Could you check a few things on this model? Use its own coordinates, in mm. A direction names the side the tool comes from. Give positions to 0.01 mm unless a question says otherwise; leave off trailing zeros. Loops run counter-clockwise (first coordinate to the right, second up) from the corner with the lowest first, then second, coordinate; pieces in that order, holes last. Notation, with made-up numbers: M -32.75,60 L -11.75,60 A26 ccw -11.75,94 Z; hole C 12,-11 d8. An arc over 180 degrees is marked long. Use a Markdown table: item, result. Add a question column.
1) Which directions (+Z, -Z, +X, -X, +Y, -Y) give clear straight access to the entire face, cutting with the end or side of a thin tool? Please do faces 1 (the cylindrical face through (190.979, -81.445, 2.535)), 2 (the cylindrical face through (131.071, -57.995, 2.465)).
2) We'd pull the mould along Y, two halves only. Please class faces 3 (the flat face through (121, -64, 0)), 4 (the cylindrical face through (8.555, -80.979, 2.535)), 5 (the flat face through (70, -72, 2)): +Y half, -Y half, draft (parallel to the pull), parting line (faces both ways), or undercut.
3) If I drill on line 1 along Y through (x, z) = (109, 2.15); line 2 along Y through (x, z) = (185, 2.5); line 3 along Y through (x, z) = (51, 1.6), over which ranges is the centre line in solid material (lowest first)? Write a range as [from, to].
4) Suppose I cut it at A-A on x = 131.5. List the corners of the cut face in (y, z) for me.
5) Suppose I cut it at D-D on y = -82.5. List the corners of the cut face in (x, z) for me.
6) Suppose I cut it at B-B on z = 2.55. Count the separate pieces of the cut face and the enclosed holes in it, and give its area (3 significant figures).
7) Suppose I cut it at C-C on x = 81. List the corners of the cut face in (y, z) for me.
```python
from build123d import *

# Parameters (mm, degrees)
SKETCH_W    = 200
SKETCH_H    = 90
SKETCH_R    = 1.5625
SKETCH_W_2  = 60
SKETCH_H_2  = 67
PAD_DEPTH   = 5
FILLET_R    = 30
FILLET001_R = 3.125
FILLET002_R = 1


with BuildPart() as part:
    # Sketch → Pad (new body)
    with BuildSketch(Plane.XY):
        with Locations((100, -45)):
            Rectangle(SKETCH_W, SKETCH_H)
        with Locations((175, -10)):
            Circle(SKETCH_R, mode=Mode.SUBTRACT)
        with Locations((175, -30)):
            Circle(SKETCH_R, mode=Mode.SUBTRACT)
        with Locations((185, -20)):
            Circle(SKETCH_R, mode=Mode.SUBTRACT)
        with Locations((185, -40)):
            Circle(SKETCH_R, mode=Mode.SUBTRACT)
        with Locations((25, -10)):
            Circle(SKETCH_R, mode=Mode.SUBTRACT)
        with Locations((25, -30)):
            Circle(SKETCH_R, mode=Mode.SUBTRACT)
        with Locations((15, -20)):
            Circle(SKETCH_R, mode=Mode.SUBTRACT)
        with Locations((15, -40)):
            Circle(SKETCH_R, mode=Mode.SUBTRACT)
        with Locations((70, -38.5)):
            Rectangle(SKETCH_W_2, SKETCH_H_2, mode=Mode.SUBTRACT)
        with BuildLine():
            ThreePointArc((158.0113, -4.9887), (155.0113, -1.9887), (152.0113, -4.9887))
            Line((152.0113, -4.9887), (152.0113, -14.9887))
            ThreePointArc((152.0113, -14.9887), (155.0113, -17.9887), (158.0113, -14.9887))
            Line((158.0113, -4.9887), (158.0113, -14.9887))
        make_face(mode=Mode.SUBTRACT)
        with BuildLine():
            ThreePointArc((151, -28.5), (131.5, -9), (112, -28.5))
            Line((112, -28.5), (112, -38.5))
            ThreePointArc((112, -38.5), (131.5, -58), (151, -38.5))
            Line((151, -28.5), (151, -38.5))
        make_face(mode=Mode.SUBTRACT)
        with BuildLine():
            ThreePointArc((158.0113, -52.0113), (155.0113, -49.0113), (152.0113, -52.0113))
            Line((152.0113, -52.0113), (152.0113, -62.0113))
            ThreePointArc((152.0113, -62.0113), (155.0113, -65.0113), (158.0113, -62.0113))
            Line((158.0113, -52.0113), (158.0113, -62.0113))
        make_face(mode=Mode.SUBTRACT)
        with BuildLine():
            ThreePointArc((110.9887, -52.0113), (107.9887, -49.0113), (104.9887, -52.0113))
            Line((104.9887, -52.0113), (104.9887, -62.0113))
            ThreePointArc((104.9887, -62.0113), (107.9887, -65.0113), (110.9887, -62.0113))
            Line((110.9887, -52.0113), (110.9887, -62.0113))
        make_face(mode=Mode.SUBTRACT)
        with BuildLine():
            ThreePointArc((110.9887, -4.9887), (107.9887, -1.9887), (104.9887, -4.9887))
            Line((104.9887, -4.9887), (104.9887, -14.9887))
            ThreePointArc((104.9887, -14.9887), (107.9887, -17.9887), (110.9887, -14.9887))
            Line((110.9887, -4.9887), (110.9887, -14.9887))
        make_face(mode=Mode.SUBTRACT)
    extrude(amount=PAD_DEPTH)

    # Fillet
    fillet_edges = [part.edges().sort_by_distance(p)[0] for p in [
        (200, -90, 2.5),
        (0, -90, 2.5),
    ]]
    fillet(fillet_edges, radius=FILLET_R)

    # Fillet001
    fillet001_edges = [part.edges().sort_by_distance(p)[0] for p in [
        (100, -5, 2.5),
        (100, -72, 2.5),
        (40, -72, 2.5),
        (40, -5, 2.5),
    ]]
    fillet(fillet001_edges, radius=FILLET001_R)

    # Fillet002
    fillet002_edges = [part.edges().sort_by_distance(p)[0] for p in [
        (200, 0, 2.5),
        (0, 0, 2.5),
    ]]
    fillet(fillet002_edges, radius=FILLET002_R)


solid = part.part
```
Answer block:
| question | item | result |
|---|---|---|
| 1 | face 1 | +Z, -Z, +X, -Y |
| 1 | face 2 | +Z, -Z |
| 2 | face 3 | draft |
| 2 | face 4 | -Y half |
| 2 | face 5 | undercut |
| 3 | line 1 | y = [-90, -64.84], [-49.19, -17.81], [-2.16, 0] |
| 3 | line 2 | y = [-85.98, -41.56], [-38.44, -21.56], [-18.44, 0] |
| 3 | line 3 | y = [-90, -72], [-5, 0] |
| 4 | outline | M -90,0 L -58,0 L -58,5 L -90,5 Z; M -9,0 L 0,0 L 0,5 L -9,5 Z |
| 5 | outline | M 10.16,0 L 189.84,0 L 189.84,5 L 10.16,5 Z |
| 6 | separate pieces | 1 |
| 6 | enclosed holes | 14 |
| 6 | area | 11,600 mm^2 |
| 7 | outline | M -90,0 L -72,0 L -72,5 L -90,5 Z; M -5,0 L 0,0 L 0,5 L -5,5 Z |
